Source: three-view drawing plus pictorial views. Frame: mm from the lowest corner of the part. Give positions to 0.01 mm unless a question says otherwise; leave off trailing zeros. Order: outer loops, then holes, each group sorted by start corner. A loop starts at its lowest first (then second) coordinate and runs counter-clockwise, first axis right, second up.
1) Section B-B, the plane z = 3.9. Return loops of the section in (x, y).
2) Section C-C, the plane x = 105. Return loops of the section in (y, z), plus the area to 3 significant figures.
3) Material intervals for line 1 (Y direction, x = 43, z = 2.5); line 2 (Y direction, x = 105, z = 2.55); line 3 (X direction, y = 40.5, z = 2.1), sorted ascending.
4) First-contact query: P1, Ø1.5, axis at y = 9.5, z = 2.5, coming from the +X side. Flat tip, straight axial feed; report the tip coordinate or a pass-through.
5) Section A-A, the plane y = 25. Return loops of the section in (x, z).
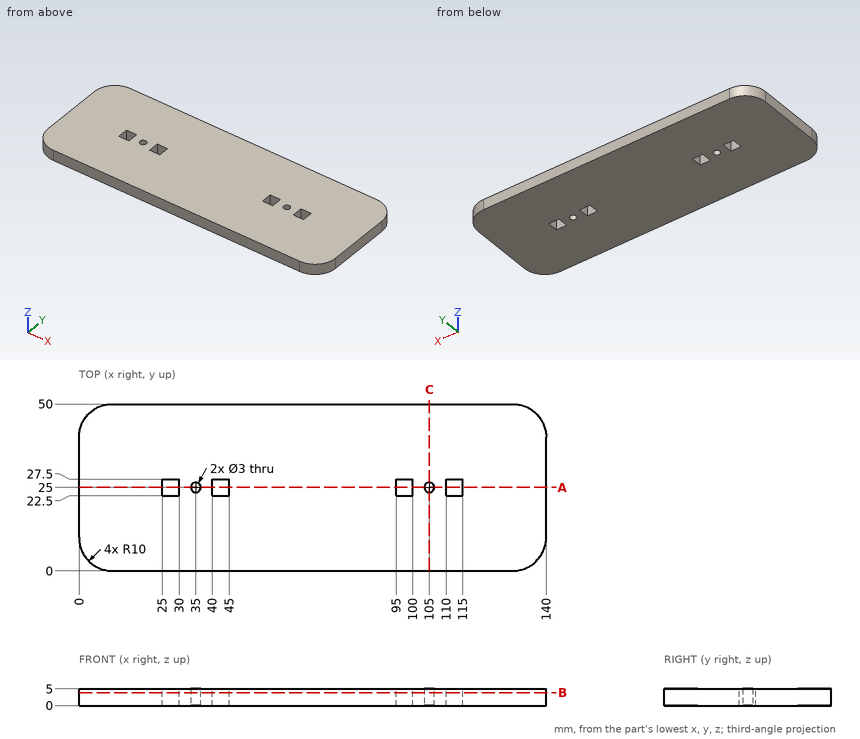
From the geometry:
1. outline: (0, 10) arc R10 ccw to (10, 0) - (130, 0) arc R10 ccw to (140, 10) - (140, 40) arc R10 ccw to (130, 50) - (10, 50) arc R10 ccw to (0, 40) - close; hole (25, 22.5) - (30, 22.5) - (30, 27.5) - (25, 27.5) - close; hole circle Ø3 at (35, 25); hole (40, 22.5) - (45, 22.5) - (45, 27.5) - (40, 27.5) - close; hole (95, 22.5) - (100, 22.5) - (100, 27.5) - (95, 27.5) - close; hole circle Ø3 at (105, 25); hole (110, 22.5) - (115, 22.5) - (115, 27.5) - (110, 27.5) - close
2. outline: (0, 0) - (23.5, 0) - (23.5, 5) - (0, 5) - close; (26.5, 0) - (50, 0) - (50, 5) - (26.5, 5) - close
2. area: 235 mm2
3. line 1: y = 0 to 22.5, 27.5 to 50
3. line 2: y = 0 to 23.5, 26.5 to 50
3. line 3: x = 0.01 to 139.99
4. P1: stops at x = 140
5. outline: (0, 0) - (25, 0) - (25, 5) - (0, 5) - close; (30, 0) - (33.5, 0) - (33.5, 5) - (30, 5) - close; (36.5, 0) - (40, 0) - (40, 5) - (36.5, 5) - close; (45, 0) - (95, 0) - (95, 5) - (45, 5) - close; (100, 0) - (103.5, 0) - (103.5, 5) - (100, 5) - close; (106.5, 0) - (110, 0) - (110, 5) - (106.5, 5) - close; (115, 0) - (140, 0) - (140, 5) - (115, 5) - close
